from build123d import *

# Parameters (mm, degrees)
F0_W     = 1828.8
F0_H     = 762
F1_DEPTH = 406.4
F3_DEPTH = 50.8
F2_W     = 1625.6
F2_H     = 406.4
F4_DEPTH = 762
F5_W     = 558.8
F5_H     = 406.4
F6_DEPTH = 1828.8


with BuildPart() as f1:
    # F0 (on Top) → F1 (new body)
    with BuildSketch(Plane.XY):
        Rectangle(F0_W, F0_H)
    extrude(amount=F1_DEPTH)

    # F3 (add): a face of the model
    f3_faces = [f1.faces().sort_by_distance(p)[0] for p in [
        (0, 0, 406.4),
    ]]
    extrude(f3_faces, amount=F3_DEPTH)

    # F2 (on face) → F4 (cut)
    with BuildSketch(Plane.XZ.offset(381)):
        with Locations((0, 203.2)):
            Rectangle(F2_W, F2_H)
    extrude(amount=-F4_DEPTH, mode=Mode.SUBTRACT)

    # F5 (on face) → F6 (cut)
    with BuildSketch(Plane.YZ.offset(914.4)):
        with Locations((0, 203.2)):
            Rectangle(F5_W, F5_H)
    extrude(amount=-F6_DEPTH, mode=Mode.SUBTRACT)


solid = f1.part
Work out the finished part from the listing and answer in its coordinate system (mm). A direction names the side the tool comes from. Round coordinates to 2 decimals unless told otherwise and drop trailing zeros. Write each loop counter-clockwise with the first axis right and the second up, starting at its lowest first coordinate (ties: lowest second). Pieces come first, ordered by that corner, then holes.
1) A cutting plane is placed at A-A (z = 217). Give the vertices of the cut face in (x, y).
2) Straight lines are drawn through the part: line 1 (X direction, y = -333, z = 303.5); line 2 (Z direction, x = 158, y = -242.5). For each, find the intervals that lie inside material, in ascending order.
3) A cutting plane is placed at B-B (x = 713.5). Give the vertices of the cut face in (y, z), plus the area to 3 significant figures.
4) A cutting plane is placed at C-C (y = 204). Give the vertices of the cut face in (x, z), plus the area to 3 significant figures.
5) Given pin 1 Ø5 at (x, y) = (-407.5, 3.5) entering from -Z, flat-ended and moving along its own axis, determine where the tip first touches the part or whether it passes through.
6) A tool of negligible diameter and unlimited length cuts with its end or side. For faces 1 (the flat face through (-812.8, -331, 200)), 2 (the flat face through (-140, -381, 414)), 3 (the flat face through (864, -279.4, 200)), from which of +Z, -Z, +X, -X, +Y, -Y can it reach the whole face along a straight path? Write none if from no direction.
Completed:
1. outline: (-914.4, -381) - (-812.8, -381) - (-812.8, -279.4) - (-914.4, -279.4) - close; (-914.4, 279.4) - (-812.8, 279.4) - (-812.8, 381) - (-914.4, 381) - close; (812.8, -381) - (914.4, -381) - (914.4, -279.4) - (812.8, -279.4) - close; (812.8, 279.4) - (914.4, 279.4) - (914.4, 381) - (812.8, 381) - close
2. line 1: x = -914.4 to -812.8, 812.8 to 914.4
2. line 2: z = 406.4 to 457.2
3. outline: (-381, 406.4) - (381, 406.4) - (381, 457.2) - (-381, 457.2) - close
3. area: 38,700 mm2
4. outline: (-914.4, 406.4) - (914.4, 406.4) - (914.4, 457.2) - (-914.4, 457.2) - close
4. area: 92,900 mm2
5. pin 1: stops at z = 406.4
6. face 1: -Z, +Y, -Y
6. face 2: +Z, -Z, +X, -X, -Y
6. face 3: -Z, +X, -X
